Autodesk Inventor part; units mm, degrees
ref_plane "YZ Plane" through (0, 0, 0) normal (1, 0, 0) x (0, 1, 0)
ref_plane "XZ Plane" through (0, 0, 0) normal (0, 1, 0) x (-1, 0, 0)
ref_plane "XY Plane" through (0, 0, 0) normal (0, 0, 1) x (1, 0, 0)
sketch "Sketch1" plane through (0, 0, 0) normal (0, 0, 1) x (1, 0, 0)
  circle A0 centre (0, 0) radius 16.5
  circle A1 centre (0, 0) radius 19.5
  dimension "d0" = 33
  dimension "d1" = 39
extrude "Extrusion1" add sketch "Sketch1" along normal blind 195
ref_plane "Work Plane1" through (0, 0, 97.5) normal (0, 0, 1) x (1, 0, 0)
sketch "Sketch2" plane through (0, 0, 195) normal (0, 0, 1) x (1, 0, 0)
  circle A0 centre (0, 0) radius 19.5
extrude "Extrusion2" add sketch "Sketch2" along normal blind 3
mirror "Mirror1" about plane through (0, 0, 97.5) normal (0, 0, 1) of "Extrusion2"
sketch "Sketch5" plane through (0, 0, -3) normal (0, 0, -1) x (-1, 0, 0)
  circle A0 centre (0, 0) radius 11
  dimension "d12" = 22
extrude "Extrusion5" cut sketch "Sketch5" against normal blind 10
sketch "Sketch6" plane through (0, 0, 0) normal (1, 0, 0) x (0, 1, 0)
  line L0 (11, -3) -> (-11, -3)
  line L1 (-11, 0) -> (11, 0)
  line L2 (11, 0) -> (-11, 0)
  line L3 (-11, 0) -> (-11, -3)
  line L4 (-11, -3) -> (11, -3)
  line L5 (11, -3) -> (11, 0)
  point P0 (0, 0)
extrude "Extrusion6" cut sketch "Sketch6" along normal through all
sketch "Sketch7" plane through (0, 0, 0) normal (1, 0, 0) x (0, 1, 0)
  line L0 (-16.5, 0) -> (16.5, 0)
  line L1 (16.5, 0) -> (-16, 0)
  line L2 (-16, 0) -> (-16, 7)
  line L3 (-16, 7) -> (16.5, 7)
  line L4 (16.5, 7) -> (16.5, 0)
  point P0 (0, 0)
  point P1 (-11, 0)
  point P2 (11, 0)
  dimension "d17" = 7
extrude "Extrusion7" cut sketch "Sketch7" along normal through all
sketch "Sketch8" plane through (0, 0, 195) normal (0, 0, -1) x (-1, 0, 0)
  circle A0 centre (0, 0) radius 10.2
  circle A1 centre (0, 0) radius 19.5
  circle A2 centre (0, 0) radius 19.5
  dimension "d20" = 20.4
extrude "Extrusion8" add sketch "Sketch8" along normal blind 5
sketch "Sketch9" plane through (0, 0, 97.5) normal (0, 0, 1) x (1, 0, 0)
  circle A0 centre (0, 0) radius 19.5
extrude "Extrusion9" cut sketch "Sketch9" against normal through all
sketch "Sketch10" plane through (0, 0, 97.5) normal (0, 0, -1) x (-1, 0, 0)
  circle A0 centre (0, 0) radius 16.5
  circle A1 centre (0, 0) radius 17.4
  dimension "d25" = 33
  dimension "d26" = 0.9
extrude "Extrusion10" cut sketch "Sketch10" against normal blind 3.1
properties part number "Magazine_Tube_1_3DPrint"
Geometry: final body of the model. Coordinates: model frame, mm. A direction names the side the tool comes from. Give positions to 0.01 mm unless a question says otherwise; leave off trailing zeros. Write each loop counter-clockwise with the first axis right and the second up, starting at its lowest first coordinate (ties: lowest second). Pieces come first, ordered by that corner, then holes. Notation, with made-up numbers: M 64.25,70.25 L 77.25,70.25 A11 cw 77.25,77.25 Z; hole C -31.75,-10.75 d10. An arc over 180 degrees is marked long. Answer in a Markdown table with one row per item. Add a question column.
(1) Section A-A on x = 0. Return loops of the section in (y, z), and give its area (3 significant figures).
(2) Section C-C on z = 109. Return loops of the section in (x, y).
(3) Mould query, pull axis Y, two halves, no side actions, for faces 3 (the cylindrical face through (-2.539, -19.334, 147.046)), 4 (the cylindrical face through (-4.707, 9.049, 192.535)), 5 (the flat face through (0, 0, 198)). Classes: +Y half, -Y half, draft (parallel to the pull), parting line (faces both ways), or undercut.
(4) First-contact query: pin 1 (10 mm diameter, centred on y = -15, z = 133.5, fed in from +X); pin 2 (22.5 mm diameter, centred on x = 2, y = 1.5, fed in from -Z); pin 3 (10 mm diameter, centred on x = 9, z = 178, fed in from -Y). Flat tips, straight axial feed; report the tip coordinate or a pass-through.
(5) Reachability of faces 1 (the flat face through (0, 0, 195)), 2 (the flat face through (-17.4, -2.8, 97.5)) from +Z, -Z, +X, -X, +Y, -Y: full face, straight path, thin tool, end or side. Return the list, or none.
(6) Section D-D on x = 12.5. Return loops of the section in (y, z), and give its area (3 significant figures).
(7) Ray query, line 1 (Y direction, x = 0, z = 191.55); line 2 (Y direction, x = 0, z = 98); line 3 (X direction, y = -0.5, z = 188.5). Return the intervals inside material, ascending.
Result set:
| question | item | result |
|---|---|---|
| 1 | outline | M -19.5,97.5 L -17.4,97.5 L -17.4,100.6 L -16.5,100.6 L -16.5,190 L -10.2,190 L -10.2,195 L 10.2,195 L 10.2,190 L 16.5,190 L 16.5,100.6 L 17.4,100.6 L 17.4,97.5 L 19.5,97.5 L 19.5,198 L -19.5,198 Z |
| 1 | area | 759 mm^2 |
| 2 | outline | C 0,0 d39; hole C 0,0 d33 |
| 3 | face 3 | parting line |
| 3 | face 4 | undercut |
| 3 | face 5 | draft |
| 4 | pin 1 | stops at x = 16.74 |
| 4 | pin 2 | stops at z = 190 |
| 4 | pin 3 | stops at y = -19.09 |
| 5 | face 1 | -Z |
| 5 | face 2 | -Z, +X, -X, +Y, -Y |
| 6 | outline | M -14.97,97.5 L -12.1,97.5 L -12.1,100.6 L -10.77,100.6 L -10.77,190 L 10.77,190 L 10.77,100.6 L 12.1,100.6 L 12.1,97.5 L 14.97,97.5 L 14.97,198 L -14.97,198 Z |
| 6 | area | 1,010 mm^2 |
| 7 | line 1 | y = -19.5 to -10.2, 10.2 to 19.5 |
| 7 | line 2 | y = -19.5 to -17.4, 17.4 to 19.5 |
| 7 | line 3 | x = -19.49 to -16.49, 16.49 to 19.49 |
